Work out the finished part from the listing and answer in its coordinate system (mm). Face numbers are marked on the shaded views. A direction names the side the tool comes from. Give positions to 0.01 mm unless a question says otherwise; leave off trailing zeros. Order: outer loops, then holes, each group sorted by start corner. A loop starts at its lowest first (then second) coordinate and runs counter-clockwise, first axis right, second up.
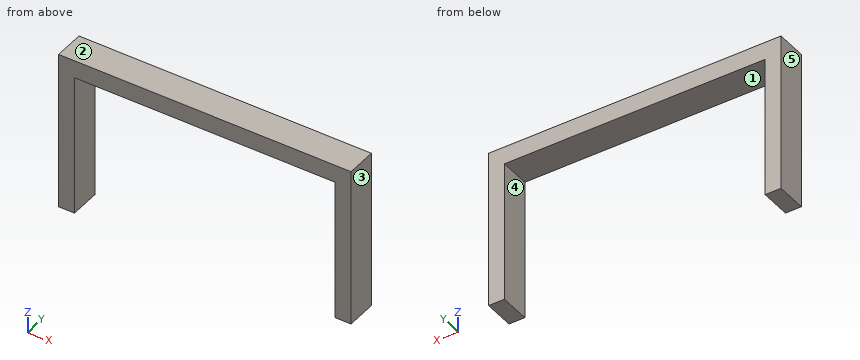
```python
from build123d import *

# Parameters (mm, degrees)
SKETCH1_W           = 2.7
SKETCH1_H           = 5.2
BOSS_EXTRUDE1_DEPTH = 27
SKETCH2_W           = 3
SKETCH2_H           = 5.2
BOSS_EXTRUDE2_DEPTH = 47
SKETCH3_W           = 2.7
SKETCH3_H           = 5.2
BOSS_EXTRUDE3_DEPTH = 24


with BuildPart() as part:
    # Sketch1 → Boss-Extrude1 (new body)
    with BuildSketch(Plane.XY):
        with Locations((1.35, 2.6)):
            Rectangle(SKETCH1_W, SKETCH1_H)
    extrude(amount=BOSS_EXTRUDE1_DEPTH)

    # Sketch2 → Boss-Extrude2 (add)
    with BuildSketch(Plane.ZY):
        with Locations((25.5, 2.6)):
            Rectangle(SKETCH2_W, SKETCH2_H)
    extrude(amount=BOSS_EXTRUDE2_DEPTH)

    # Sketch3 → Boss-Extrude3 (add)
    with BuildSketch(Plane(origin=(0, 0, 24), x_dir=(-1, 0, 0), z_dir=(0, 0, -1))):
        with Locations((45.65, 2.6)):
            Rectangle(SKETCH3_W, SKETCH3_H)
    extrude(amount=BOSS_EXTRUDE3_DEPTH)


solid = part.part
```
1. The part is cut by section B-B (y = 2.35). Write down the section's boundary in (x, z), then the cut area to 3 significant figures.
Findings below:
outline: (-47, 0) - (-44.3, 0) - (-44.3, 24) - (0, 24) - (0, 0) - (2.7, 0) - (2.7, 27) - (-47, 27) - close
area: 279 mm2
2. The part is cut by section C-C (x = -19). Write down the section's boundary in (y, z).
Findings below:
outline: (0, 24) - (5.2, 24) - (5.2, 27) - (0, 27) - close
3. The mould has two halves that part along X. Classify the marked faces 3, 4 and 5: pulls with the +X half, pulls with the -X half, needs draft (parallel to the pull), parting line crosses it, or undercut.
Findings below:
face 3: pulls with the +X half
face 4: undercut
face 5: pulls with the -X half
4. Given P1, Ø1.6, axis at x = -18, y = 1.5, coming from the -Z side; P2, Ø6, axis at x = -13.5, z = 19.5, coming from the +Y side, each flat-ended and moving along its own axis, determine where each tip first touches the part or whether it passes through.
Findings below:
P1: stops at z = 24
P2: passes through
5. Which of the six approach directions +Z, -Z, +X, -X, +Y, -Y give full straight-line access (tool end or side, diameter ignored) to the marked faces 1 and 2?
Findings below:
face 1: -Z, +Y, -Y
face 2: +Z, +X, -X, +Y, -Y
6. Straight lines are drawn through the part: probe 1 along X at (y, z) = (4.9, 14); probe 2 along Z at (x, y) = (-27, 1). For each, find the intervals that lie inside material, in ascending order.
Findings below:
probe 1: x = -47 to -44.3, 0 to 2.7
probe 2: z = 24 to 27
7. The part is cut by section A-A (z = 14.25). Write down the section's boundary in (x, y), then the cut area to 3 significant figures.
Findings below:
outline: (-47, 0) - (-44.3, 0) - (-44.3, 5.2) - (-47, 5.2) - close; (0, 0) - (2.7, 0) - (2.7, 5.2) - (0, 5.2) - close
area: 28.1 mm2
